Autodesk Inventor part; units mm, degrees
ref_plane "YZ Plane" through (0, 0, 0) normal (1, 0, 0) x (0, 1, 0)
ref_plane "XZ Plane" through (0, 0, 0) normal (0, 1, 0) x (-1, 0, 0)
ref_plane "XY Plane" through (0, 0, 0) normal (0, 0, 1) x (1, 0, 0)
sketch "Sketch1" plane through (0, 0, 0) normal (0, 0, 1) x (1, 0, 0)
  line L0 (-3.9007, 3.9007) -> (3.9007, 3.9007)
  line L1 (3.9007, 3.9007) -> (3.9007, -3.9007)
  line L2 (3.9007, -3.9007) -> (-3.9007, -3.9007)
  line L3 (-3.9007, -3.9007) -> (-3.9007, 3.9007)
  line L4 (0, 3.9007) -> (0, -3.9007) construction
  line L5 (-3.9007, 0) -> (3.9007, 0) construction
  circle A0 centre (0, 0) radius 2.1
  line L6 (0, 0) -> (-16.1173, 16.1173) construction
  line L7 (0, 0) -> (22.7933, 0) construction
  line L8 (-2.84, 3.9007) -> (-5.4993, 6.56)
  line L9 (-5.4993, 6.56) -> (-5.4993, 8.2)
  line L10 (-5.4993, 8.2) -> (-2.84, 8.2)
  line L11 (-2.84, 8.2) -> (-4.64, 10)
  line L12 (-4.64, 10) -> (-10, 10)
  line L13 (-10, 10) -> (-10, 4.64)
  line L14 (-10, 4.64) -> (-8.2, 2.84)
  line L15 (-8.2, 2.84) -> (-8.2, 5.4993)
  line L16 (-8.2, 5.4993) -> (-6.56, 5.4993)
  line L17 (-6.56, 5.4993) -> (-3.9007, 2.84)
  line L18 (-3.9007, 2.84) -> (-11.3102, 2.84) construction
  line L19 (-2.84, 3.9007) -> (-3.9007, 3.9007)
  line L20 (-3.9007, 2.84) -> (-3.9007, 3.9007)
  line L21 (-3.9007, -2.84) -> (-6.56, -5.4993)
  line L22 (-6.56, -5.4993) -> (-8.2, -5.4993)
  line L23 (-8.2, -5.4993) -> (-8.2, -2.84)
  line L24 (-8.2, -2.84) -> (-10, -4.64)
  line L25 (-10, -4.64) -> (-10, -10)
  line L26 (-10, -10) -> (-4.64, -10)
  line L27 (-4.64, -10) -> (-2.84, -8.2)
  line L28 (-2.84, -8.2) -> (-5.4993, -8.2)
  line L29 (-5.4993, -8.2) -> (-5.4993, -6.56)
  line L30 (-5.4993, -6.56) -> (-2.84, -3.9007)
  line L31 (-3.9007, -2.84) -> (-3.9007, -3.9007)
  line L32 (-2.84, -3.9007) -> (-3.9007, -3.9007)
  line L33 (2.84, -3.9007) -> (5.4993, -6.56)
  line L34 (5.4993, -6.56) -> (5.4993, -8.2)
  line L35 (5.4993, -8.2) -> (2.84, -8.2)
  line L36 (2.84, -8.2) -> (4.64, -10)
  line L37 (4.64, -10) -> (10, -10)
  line L38 (10, -10) -> (10, -4.64)
  line L39 (10, -4.64) -> (8.2, -2.84)
  line L40 (8.2, -2.84) -> (8.2, -5.4993)
  line L41 (8.2, -5.4993) -> (6.56, -5.4993)
  line L42 (6.56, -5.4993) -> (3.9007, -2.84)
  line L43 (2.84, -3.9007) -> (3.9007, -3.9007)
  line L44 (3.9007, -2.84) -> (3.9007, -3.9007)
  line L45 (3.9007, 2.84) -> (6.56, 5.4993)
  line L46 (6.56, 5.4993) -> (8.2, 5.4993)
  line L47 (8.2, 5.4993) -> (8.2, 2.84)
  line L48 (8.2, 2.84) -> (10, 4.64)
  line L49 (10, 4.64) -> (10, 10)
  line L50 (10, 10) -> (4.64, 10)
  line L51 (4.64, 10) -> (2.84, 8.2)
  line L52 (2.84, 8.2) -> (5.4993, 8.2)
  line L53 (5.4993, 8.2) -> (5.4993, 6.56)
  line L54 (5.4993, 6.56) -> (2.84, 3.9007)
  line L55 (3.9007, 2.84) -> (3.9007, 3.9007)
  line L56 (2.84, 3.9007) -> (3.9007, 3.9007)
  dimension "d7" = 4.2
  dimension "d8" = 135
  dimension "d9" = 1.5
  dimension "d10" = 1.64
  dimension "d11" = 1.8
  dimension "d12" = 2.84
  dimension "d13" = 10
  dimension "d16" = 360
extrude "Extrusion1" add sketch "Sketch1" along normal blind 150
properties part number "20x20x250mm" material "Aluminum 6061"
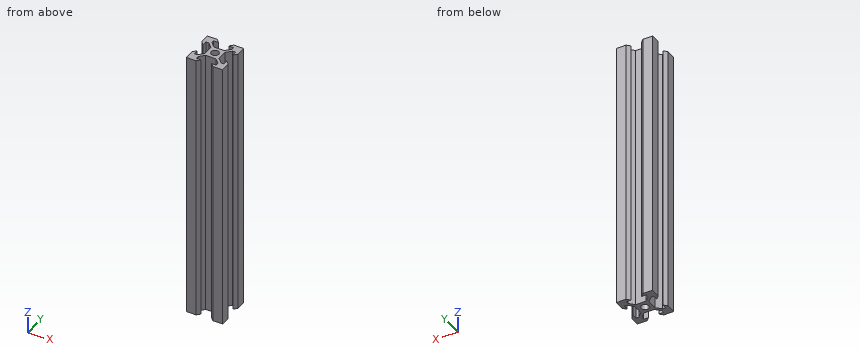
Part model, mm, in its own coordinate system. Round coordinates to 2 decimals unless told otherwise and drop trailing zeros. Order: outer loops, then holes, each group sorted by start corner. A loop starts at its lowest first (then second) coordinate and runs counter-clockwise, first axis right, second up. Notation, with made-up numbers: M 29.25,-12 L 71.25,-12 A32 cw 71.25,22 Z; hole C 46.25,27.5 d7. An arc over 180 degrees is marked long. Put each result on its own line as item: value. Start each with the question number.
1. Drop flat-ended pins along their axis: pin 1 (0.8 mm diameter, centred on x = -4, z = 95.5, fed in from -Y); pin 2 (1.7 mm diameter, centred on y = 0, z = 100, fed in from -X); pin 3 (0.8 mm diameter, centred on x = 4, z = 64.5, fed in from +Y). Give the stop position or say it passes through.
2. Slice it at A-A on y = 0. List the corners of the cut face in (x, z), then the cut area to 3 significant figures.
3. Drill centre lines: probe 1 along Y at (x, z) = (0, 44.5); probe 2 along Y at (x, z) = (7, 110); probe 3 along Y at (x, z) = (-5.25, 143.5). Where is each one in solid material? Low to high. Write a range as [from, to].
Findings:
1. pin 1: y = -9.76
1. pin 2: x = -3.9
1. pin 3: y = 9.76
2. outline: M -3.9,0 L -2.1,0 L -2.1,150 L -3.9,150 Z; M 2.1,0 L 3.9,0 L 3.9,150 L 2.1,150 Z
2. area: 540 mm2
3. probe 1: [-3.9, -2.1], [2.1, 3.9]
3. probe 2: [-10, -5.5], [5.5, 10]
3. probe 3: [-10, -8.2], [-6.31, -4.19], [4.19, 6.31], [8.2, 10]
